```python
from build123d import *

# Parameters (mm, degrees)
SKETCH1_R           = 10
BOSS_EXTRUDE1_DEPTH = 100
SKETCH4_W           = 20
SKETCH4_H           = 25
CUT_EXTRUDE2_DEPTH  = 10
FILLET3_R           = 5
SKETCH3_R           = 5
BOSS_EXTRUDE3_DEPTH = 5
SKETCH7_R           = 5
CUT_EXTRUDE3_DEPTH  = 5


with BuildPart() as part:
    # Sketch1 → Boss-Extrude1 (new body)
    with BuildSketch(Plane(origin=(0, 0, 0), x_dir=(1, 0, 0), z_dir=(0, 1, 0))):
        with Locations(Location((0, 0, 0), (0, 0, 90))):
            Circle(SKETCH1_R)
    extrude(amount=BOSS_EXTRUDE1_DEPTH)

    # Sketch4 → Cut-Extrude2 (cut)
    with BuildSketch(Plane.XY):
        with Locations((0, 87.5)):
            Rectangle(SKETCH4_W, SKETCH4_H)
    extrude(amount=-CUT_EXTRUDE2_DEPTH, mode=Mode.SUBTRACT)

    # Fillet3
    fillet3_edges = [part.edges().sort_by_distance(p)[0] for p in [
        (0, 100, 0),
        (0, 100, 10),
    ]]
    fillet(fillet3_edges, radius=FILLET3_R - 0.0001)  # a hair under: the kernel refuses the full size

    # Sketch3 → Boss-Extrude3 (add)
    with BuildSketch(Plane(origin=(0, 0, 0), x_dir=(1, 0, 0), z_dir=(0, 1, 0))):
        with Locations(Location((0, 0, 0), (0, 0, 270))):
            Circle(SKETCH3_R)
    extrude(amount=-BOSS_EXTRUDE3_DEPTH)

    # Sketch7 → Cut-Extrude3 (cut)
    with BuildSketch(Plane.XY):
        with Locations(Location((0, 92.001790993, 0), (0, 0, 143.155752141))):
            Circle(SKETCH7_R)
    extrude(amount=CUT_EXTRUDE3_DEPTH, mode=Mode.SUBTRACT)


solid = part.part
```
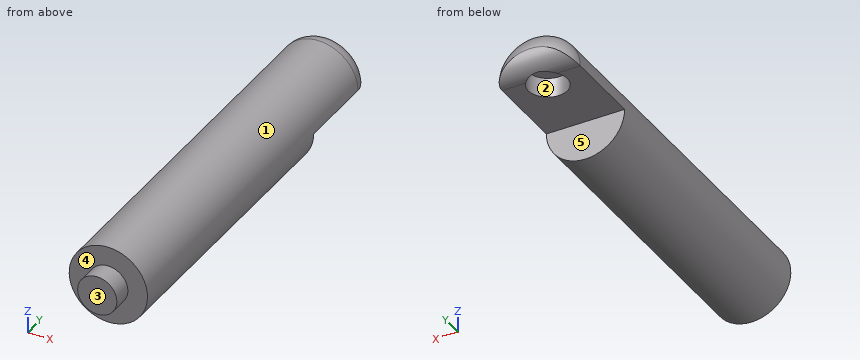
Can you work these out from the model? Positions are in its coordinate system, mm. Face numbers are marked on the shaded views. A direction names the side the tool comes from. Coordinates: 2 decimals unless noted, no trailing zeros. Write each loop counter-clockwise with the first axis right and the second up, starting at its lowest first coordinate (ties: lowest second). Pieces come first, ordered by that corner, then holes. Notation, with made-up numbers: M -3.75,45.5 L 17.25,45.5 A27 ccw 17.25,72.5 Z; hole C 29,28 d9. An arc over 180 degrees is marked long. Answer as CSV lines item,"result".
Item 1: On a 3-axis mill with a long thin cutter (end or side, diameter ignored), from which of +Z, -Z, +X, -X, +Y, -Y can I reach the whole of each face in a straight line? I mean the marked faces 4 and 5. Say none if no direction works.
Geometry results:
face 4,"-Y"
face 5,"-Z, +X, -X, +Y"
Item 2: Imagine slicing it at C-C on y = 77.5. List the corners of the cut face in (x, z) for me.
Geometry results:
outline,"M -10,0 L 10,0 A10 ccw Z"
Item 3: We'd pull the mould along X, two halves only. Please class the marked faces 1, 2 and 3: +X half, -X half, draft (parallel to the pull), parting line (faces both ways), or undercut.
Geometry results:
face 1,"parting line"
face 2,"undercut"
face 3,"draft"
Item 4: Imagine slicing it at D-D on z = -7.25. List the corners of the cut face in (x, y) for me.
Geometry results:
outline,"M -6.89,0 L 6.89,0 L 6.89,75 L -6.89,75 Z"
Item 5: I'm going to push flat-ended pins straight in: P1, Ø4, axis at x = -5, y = 43.5, coming from the -Z side; P2, Ø4, axis at y = 62, z = -7.5, coming from the -X side; P3, Ø6, axis at x = 4, z = 1.5, coming from the +Y side; P4, Ø5, axis at y = 64.5, z = -2, coming from the +X side. Where does each tip first touch, or does it pass through?
Geometry results:
P1,"stops at z = -9.54"
P2,"stops at x = -8.35"
P3,"stops at y = 99.97"
P4,"stops at x = 10"
Item 6: Please list where these lines run through material, in increasing order: line 1 along Y through (x, z) = (-8.25, -5); line 2 along Z through (x, y) = (-0.25, 28); line 3 along Y through (x, z) = (0, 2.2).
Geometry results:
line 1,"y = 0 to 75"
line 2,"z = -10 to 10"
line 3,"y = -5 to 87, 97 to 99.14"
Item 7: Imagine slicing it at B-B on y = 54. List the corners of the cut face in (x, z) for me.
Geometry results:
outline,"C 0,0 d20"
Item 8: Imagine slicing it at A-A on z = -1.75. List the corners of the cut face in (x, y) for me.
Geometry results:
outline,"M -9.85,0 L -4.68,0 L -4.68,-5 L 4.68,-5 L 4.68,0 L 9.85,0 L 9.85,75 L -9.85,75 Z"
